Read the model definition and answer for the solid it produces. Units are mm, in the model's axes. A direction names the side the tool comes from. Give positions to 0.01 mm unless a question says otherwise; leave off trailing zeros. Order: outer loops, then holes, each group sorted by start corner. A loop starts at its lowest first (then second) coordinate and runs counter-clockwise, first axis right, second up. Notation, with made-up numbers: M -10,55.25 L -6,55.25 A13 cw -6,70.25 Z; hole C 12.5,11.25 d9. An arc over 180 degrees is marked long. One line per item, written item: value.
from build123d import *

# Parameters (mm, degrees)
SKETCH1_R                            = 12.7
BOSS_EXTRUDE2_DEPTH                  = 304.8
BOSS_EXTRUDE2_2_DEPTH                = 304.8
SKETCH10_R                           = 11.43
CUT_EXTRUDE1_DEPTH                   = 304.8
SKETCH11_R                           = 11.43
BOSS_EXTRUDE3_DEPTH                  = 5.08
SKETCH12_R                           = 11.43
BOSS_EXTRUDE4_DEPTH                  = 5.08
CUT_EXTRUDE2_DEPTH                   = 13.97
SKETCH14_R                           = 11.43
CUT_EXTRUDE3_DEPTH                   = 299.72
BOSS_EXTRUDE5_REACH                  = 316.437
BOSS_EXTRUDE5_END_RADIUS             = 12.7
SKETCH15_R                           = 10.16
BOSS_EXTRUDE5_DIRECTION_2_REACH      = 316.437
BOSS_EXTRUDE5_DIRECTION_2_END_RADIUS = 12.7
CUT_EXTRUDE4_REACH                   = 337.53
CUT_EXTRUDE4_END_RADIUS              = 11.43
SKETCH17_R                           = 8.89


with BuildPart() as part:
    # Sketch1 → Boss-Extrude2 (new body)
    with BuildSketch(Plane.XY):
        with Locations(Location((0, 0, 0), (0, 0, 180))):
            Circle(SKETCH1_R)
    extrude(amount=BOSS_EXTRUDE2_DEPTH)

    # Sketch10 → Cut-Extrude1 (cut)
    with BuildSketch(Plane(origin=(0, 0, 0), x_dir=(-1, 0, 0), z_dir=(0, 0, -1))):
        Circle(SKETCH10_R)
    extrude(amount=-CUT_EXTRUDE1_DEPTH, mode=Mode.SUBTRACT)

    # Sketch11 → Boss-Extrude3 (add)
    with BuildSketch(Plane(origin=(0, 0, 0), x_dir=(-1, 0, 0), z_dir=(0, 0, -1))):
        Circle(SKETCH11_R)
    extrude(amount=-BOSS_EXTRUDE3_DEPTH)

    # Sketch12 → Boss-Extrude4 (add)
    with BuildSketch(Plane.XY.offset(304.8)):
        with Locations(Location((0, 0, 0), (0, 0, 180))):
            Circle(SKETCH12_R)
    extrude(amount=-BOSS_EXTRUDE4_DEPTH)

    # Sketch3 → Cut-Extrude2 (cut, symmetric)
    with BuildSketch(Plane(origin=(0, 0, 0), x_dir=(1, 0, 0), z_dir=(0, 1, 0))):
        Polygon((12.7, -12.7), (0, -12.7), (12.7, -25.4), align=None)
    extrude(amount=CUT_EXTRUDE2_DEPTH, both=True, mode=Mode.SUBTRACT)



with BuildPart() as body_2:
    # Sketch1 → Boss-Extrude2 2 (new body)
    with BuildSketch(Plane.XY):
        with Locations(Location((127, 0, 0), (0, 0, 180))):
            Circle(SKETCH1_R)
    extrude(amount=BOSS_EXTRUDE2_2_DEPTH)

    # Sketch14 → Cut-Extrude3 (cut)
    with BuildSketch(Plane(origin=(0, 0, 0), x_dir=(-1, 0, 0), z_dir=(0, 0, -1))):
        with Locations((-127, 0)):
            Circle(SKETCH14_R)
    extrude(amount=-CUT_EXTRUDE3_DEPTH, mode=Mode.SUBTRACT)


with BuildPart() as part_1:
    add(part.part)

    add(body_2.part)  # Boss-Extrude5 merges body 2
    # Boss-Extrude5: up to this cylinder (the profile starts outside it)
    boss_extrude5_end = Plane(origin=(127, 0, 254), z_dir=(0, 0, -1)) * Cylinder(BOSS_EXTRUDE5_END_RADIUS, 659.274, mode=Mode.PRIVATE)
    # Sketch15 → Boss-Extrude5 (add, up to the surface)
    with BuildSketch(Plane(origin=(63.5, 0, 0), x_dir=(0, 0, -1), z_dir=(1, 0, 0)), mode=Mode.PRIVATE) as boss_extrude5_sk1:
        with Locations(Location((-254, 0, 0), (0, 0, 180))):
            Circle(SKETCH15_R)
    boss_extrude5_tool1 = extrude(boss_extrude5_sk1.sketch, amount=BOSS_EXTRUDE5_REACH, mode=Mode.PRIVATE) - boss_extrude5_end
    add(boss_extrude5_tool1.solids().sort_by_distance((63.5, 0, 254))[0])

    # Boss-Extrude5 direction 2: up to this cylinder (the profile starts outside it)
    boss_extrude5_direction_2_end = Plane(origin=(0, 0, 254), z_dir=(0, 0, -1)) * Cylinder(BOSS_EXTRUDE5_DIRECTION_2_END_RADIUS, 659.274, mode=Mode.PRIVATE)
    # Sketch15 → Boss-Extrude5 direction 2 (add, up to the surface)
    with BuildSketch(Plane(origin=(63.5, 0, 0), x_dir=(0, 0, -1), z_dir=(1, 0, 0)), mode=Mode.PRIVATE) as boss_extrude5_direction_2_sk1:
        with Locations(Location((-254, 0, 0), (0, 0, 180))):
            Circle(SKETCH15_R)
    boss_extrude5_direction_2_tool1 = extrude(boss_extrude5_direction_2_sk1.sketch, amount=-BOSS_EXTRUDE5_DIRECTION_2_REACH, mode=Mode.PRIVATE) - boss_extrude5_direction_2_end
    add(boss_extrude5_direction_2_tool1.solids().sort_by_distance((63.5, 0, 254))[0])

    # Cut-Extrude4: up to this cylinder (the profile starts outside it)
    cut_extrude4_end = Plane(origin=(127, 0, 254), z_dir=(0, 0, -1)) * Cylinder(CUT_EXTRUDE4_END_RADIUS, 698.92, mode=Mode.PRIVATE)
    # Sketch17 → Cut-Extrude4 (cut, up to the surface)
    with BuildSketch(Plane(origin=(0, 0, 0), x_dir=(0, 0, -1), z_dir=(1, 0, 0)), mode=Mode.PRIVATE) as cut_extrude4_sk1:
        with Locations(Location((-254, 0, 0), (0, 0, 180))):
            Circle(SKETCH17_R)
    cut_extrude4_tool1 = extrude(cut_extrude4_sk1.sketch, amount=CUT_EXTRUDE4_REACH, mode=Mode.PRIVATE) - cut_extrude4_end
    add(cut_extrude4_tool1.solids().sort_by_distance((0, 0, 254))[0], mode=Mode.SUBTRACT)


solid = part_1.part
1) Find section D-D, the plane x = 70.5. Write down the section's boundary in (y, z).
Reported:
outline: C 0,254 d20.32; hole C 0,254 d17.78
2) Determine the mould class of faces 4 (the face through (127, 0, 304.8)), 5 (the face through (127, 0, 299.72)), 6 (the face through (139.688, -0.558, 150.266)) for opening direction Y: +Y half, -Y half, draft (parallel to the pull), parting line (faces both ways), or undercut.
Reported:
face 4: draft
face 5: undercut
face 6: parting line
3) Which of the six approach directions +Z, -Z, +X, -X, +Y, -Y give full straight-line access (tool end or side, diameter ignored) to faces 1 (the face through (0, 0, 304.8)), 2 (the face through (138.42, 0.5, 147.76)), 3 (the face through (0, 0, 5.08))?
Reported:
face 1: +Z, +X, -X, +Y, -Y
face 2: -Z
face 3: none
4) Find section B-B, the plane y = 0. Write down the section's boundary in (x, z), plus the area to 3 significant figures.
Reported:
outline: M -12.7,0 L 12.7,0 L 12.7,12.7 L 11.43,12.7 L 11.43,5.08 L -11.43,5.08 L -11.43,299.72 L 11.43,299.72 L 11.43,262.89 L 115.57,262.89 L 115.57,299.72 L 138.43,299.72 L 138.43,0 L 139.7,0 L 139.7,304.8 L 114.3,304.8 L 114.3,264.16 L 12.7,264.16 L 12.7,304.8 L -12.7,304.8 Z; M 11.43,24.13 L 12.7,25.4 L 12.7,243.84 L 114.3,243.84 L 114.3,0 L 115.57,0 L 115.57,245.11 L 11.43,245.11 Z
area: 2,090 mm^2
5) Find section C-C, the plane z = 153. Write down the section's boundary in (x, y).
Reported:
outline: C 0,0 d25.4; C 127,0 d25.4; hole C 0,0 d22.86; hole C 127,0 d22.86
6) Find section A-A, the plane z = 254. Write down the section's boundary in (x, y), plus the area to 3 significant figures.
Reported:
outline: M 7.62,-10.16 L 119.38,-10.16 A12.7 ccw long 119.38,10.16 L 7.62,10.16 A12.7 ccw long Z; hole M 7.18,-8.89 L 119.82,-8.89 A11.43 ccw long 119.82,8.89 L 7.18,8.89 A11.43 ccw long Z
area: 422 mm^2
7) Consider probe 1 along X at (y, z) = (0.5, 99); probe 2 along Y at (x, z) = (127, 226.5); probe 3 along X at (y, z) = (-4, 34.5). Determine where each line is inside the solid, lowest interval first.
Reported:
probe 1: x = -12.69 to -11.42, 11.42 to 12.69, 114.31 to 115.58, 138.42 to 139.69
probe 2: y = -12.7 to -11.43, 11.43 to 12.7
probe 3: x = -12.05 to -10.71, 10.71 to 12.05, 114.95 to 116.29, 137.71 to 139.05
8) Each of these flat-tipped pins is pushed along its axis until it touches: pin 1 Ø6 at (y, z) = (6.5, 179) entering from -X; pin 2 Ø12 at (x, y) = (86, -8.5) entering from -Z; pin 3 Ø1.5 at (x, z) = (116, 234) entering from +Y; pin 4 Ø6 at (x, z) = (110.5, 86.5) entering from -Y. Where does it stop, or does it pass through?
Reported:
pin 1: stops at x = -12.21
pin 2: stops at z = 244.15
pin 3: stops at y = 7.5
pin 4: passes through
